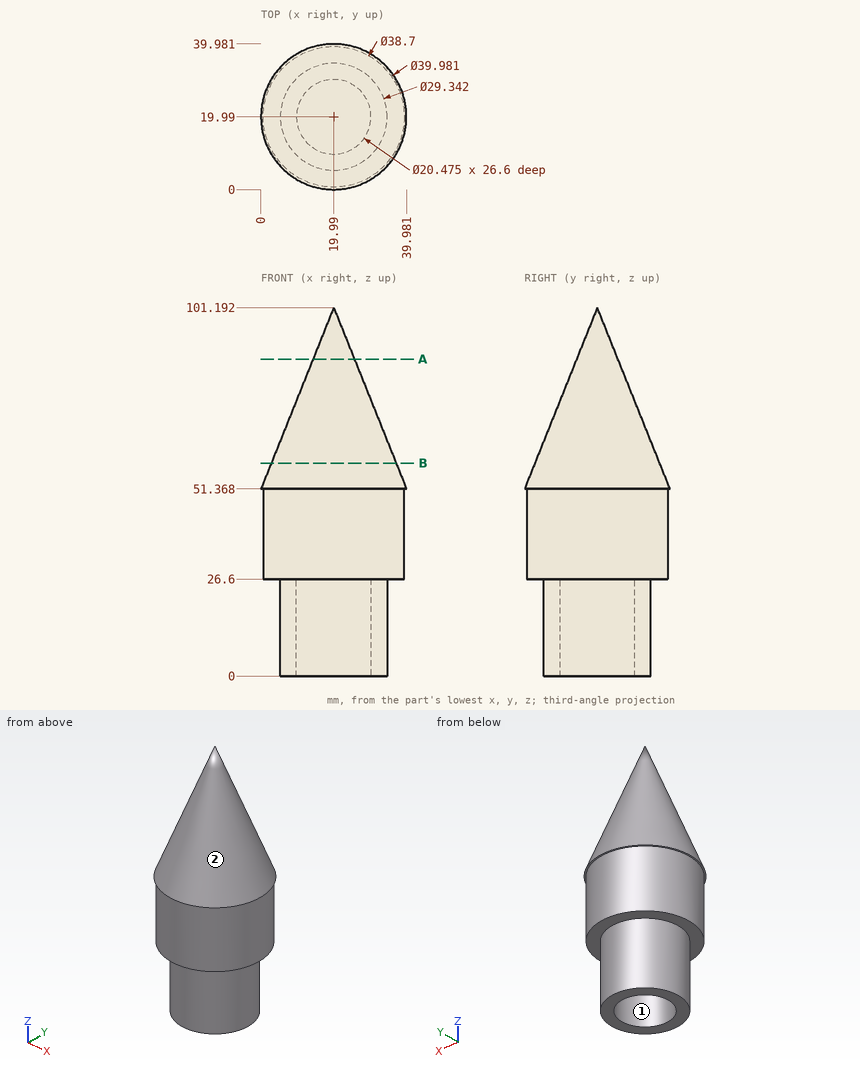
The drawing under review shows one solid part. Ordinate dimensions are in mm from its lowest x, y, z. Give positions to 0.01 mm unless a question says otherwise; leave off trailing zeros. Order: outer loops, then holes, each group sorted by start corner. A loop starts at its lowest first (then second) coordinate and runs counter-clockwise, first axis right, second up. Notation, with made-up numbers: (-29.75, -6) -> (13.25, -6) arc R24 cw to (13.25, 30) -> close; hole circle Ø5 at (55.25, 29.25). An arc over 180 degrees is marked (long way). Write item = value, one per line. Start each with the question number.
(1) We need section A-A on z = 87. Write out the cut boundary in (x, y) (1 decimal).
(2) To check wall thickness, follow line 1 along X through (y, z) = (18.5, 24.5) (1 decimal); line 2 along Y through (x, z) = (24, 61.5); line 3 along Y through (x, z) = (32, 24) (1 decimal). State the ranges of each line that lie inside material, in increasing order.
(3) Mouldability with a two-part tool opening along Y and no side actions: class the marked faces 1 and 2 as +Y half, -Y half, draft (parallel to the pull), parting line (faces both ways), or undercut.
(4) We need section B-B on z = 58.5. Write out the cut boundary in (x, y).
(5) For pin 1 (8 mm diameter, centred on y = 33, z = 75, fed in from -X); pin 2 (1 mm diameter, centred on y = 20, z = 27.5, fed in from -X); pin 3 (6 mm diameter, centred on x = 23.5, y = 21, fed in from -Z), all flat-tipped, find the tip position at first contact; note any pin that passes through.
Numbers:
q1.outline = circle Ø11.4 at (20, 20)
q2.line_1 = 5.4 to 9.9, 30.1 to 34.6
q2.line_2 = 4.58 to 35.4
q2.line_3 = 11.6 to 28.4
q3.face_1 = undercut
q3.face_2 = parting line
q4.outline = circle Ø34.26 at (19.99, 19.99)
q5.pin_1 = 13.9
q5.pin_2 = 0.64
q5.pin_3 = 26.6
